```python
from build123d import *

# Parameters (mm, degrees)
PAD_DEPTH         = 20
SKETCH002_R       = 2
POCKET_DEPTH      = 20.143136
POCKET_DEPTH_BACK = 44.001
SKETCH003_R       = 4
POCKET001_DEPTH   = 44.001
CHAMFER_SIZE2     = 1.9999
CHAMFER_SIZE      = 3
FILLET_R          = 5


with BuildPart() as part:
    # Sketch → Pad (new body)
    with BuildSketch(Plane.XY):
        Polygon((0, 0), (50.710678, 0), (70.710678, 20), (0, 20), align=None)
    extrude(amount=PAD_DEPTH)

    # Sketch002 (on DatumPlane) → Pocket (cut, two sides)
    with BuildSketch(Plane(origin=(21.112698, -21.112698, 0), x_dir=(-0.707107, -0.707107, 0), z_dir=(-0.707107, 0.707107, 0))) as pocket_sk:
        with Locations((-50, 10)):
            Circle(SKETCH002_R)
    extrude(amount=-POCKET_DEPTH, mode=Mode.SUBTRACT)
    extrude(pocket_sk.sketch, amount=POCKET_DEPTH_BACK, mode=Mode.SUBTRACT)

    # Sketch003 (on DatumPlane) → Pocket001 (cut, through all)
    with BuildSketch(Plane(origin=(21.112698, -21.112698, 0), x_dir=(-0.707107, -0.707107, 0), z_dir=(-0.707107, 0.707107, 0))):
        with Locations((-50, 10)):
            Circle(SKETCH003_R)
    extrude(amount=POCKET001_DEPTH, mode=Mode.SUBTRACT)

    # Chamfer
    chamfer_edges = [part.edges().sort_by_distance(p)[0] for p in [
        (57.882251, 15.656854, 10),
    ]]
    chamfer_side = part.faces().sort_by_distance((60.003571, 13.535534, 10))[0]
    chamfer(chamfer_edges, length=CHAMFER_SIZE, length2=CHAMFER_SIZE2, reference=chamfer_side)

    # Fillet
    fillet_edges = [part.edges().sort_by_distance(p)[0] for p in [
        (35.355339, 20, 20),
        (25.355339, 0, 20),
        (35.355339, 20, 0),
        (25.355339, 0, 0),
    ]]
    fillet(fillet_edges, radius=FILLET_R)

    # Mirrored: part across YZ


with BuildPart() as part_1:
    add(part.part)
    add(part.part.mirror(Plane.YZ))


solid = part_1.part
```
Here's how the part is built. I have some questions about the finished solid (model axes, mm). Round coordinates to 2 decimals unless told otherwise and drop trailing zeros. Order: outer loops, then holes, each group sorted by start corner. A loop starts at its lowest first (then second) coordinate and runs counter-clockwise, first axis right, second up. Notation, with made-up numbers: (40.5, 87.5) -> (51.5, 87.5) arc R10 ccw to (51.5, 101.5) -> close; hole circle Ø8 at (-14.75, -23.75). An arc over 180 degrees is marked (long way). Use a Markdown table: item, result. Add a question column.
(1) Suppose I cut it at B-B, the plane z = 18.25. Please give me the cut outline in (x, y).
(2) For pin 1 Ø8 at (y, z) = (6, 15) entering from -X; pin 2 Ø1 at (x, z) = (53, 17.5) entering from -Y; pin 3 Ø3 at (x, z) = (-56, 9) entering from -Y, each with a flat end and sliding along its axis, tell me the tip position at first contact or that it passes through.
(3) If we mould it in two halves opening along Z, with no side actions, what happens to faces 1 (the face through (-1, 1, 2)), 2 (the face through (59.958, 13.755, 10.093)), 3 (the face through (1, 18, 19))? For each: released by +Z, released by -Z, zero draft, split by the parting line, or undercut.
(4) Suppose I cut it at A-A, the plane x = 17. Please give me the cut outline in (y, z), and give its area (3 significant figures).
(5) Suppose I cut it at C-C, the plane y = 7. Please give me the cut outline in (x, z), and give its area (3 significant figures).
(6) I need wall thicknesses on line 1 along X through (y, z) = (18.25, 13.25); line 2 along X through (y, z) = (16.5, 11.25); line 3 along X through (y, z) = (1.75, 7.25). Which ranges of each line are inside material? Lowest first, please.
Verdict:
| question | item | result |
|---|---|---|
| 1 | outline | (-69.51, 18.8) -> (-51.91, 1.2) -> (51.91, 1.2) -> (69.51, 18.8) -> close |
| 2 | pin 1 | x = -60.71 |
| 2 | pin 2 | y = 1.79 |
| 2 | pin 3 | y = 3.79 |
| 3 | face 1 | released by -Z |
| 3 | face 2 | undercut |
| 3 | face 3 | released by +Z |
| 4 | outline | (0, 5) arc R5 ccw to (5, 0) -> (15, 0) arc R5 ccw to (20, 5) -> (20, 15) arc R5 ccw to (15, 20) -> (5, 20) arc R5 ccw to (0, 15) -> close |
| 4 | area | 379 mm2 |
| 5 | outline | (-57.71, 0) -> (57.71, 0) -> (57.71, 20) -> (-57.71, 20) -> close |
| 5 | area | 2,310 mm2 |
| 6 | line 1 | -68.96 to -55.76, -49.16 to 49.16, 55.76 to 68.96 |
| 6 | line 2 | -67.21 to -59.23, -48.84 to 48.84, 59.23 to 67.21 |
| 6 | line 3 | -52.46 to 52.46 |
